For this review, take the finished solid that the model builds, in its own axes (mm). Face numbers are marked on the shaded views. A direction names the side the tool comes from. Give positions to 0.01 mm unless a question says otherwise; leave off trailing zeros. Order: outer loops, then holes, each group sorted by start corner. A loop starts at its lowest first (then second) coordinate and runs counter-clockwise, first axis right, second up. Notation, with made-up numbers: M -38,82.5 L -9,82.5 A31 ccw -9,112.5 Z; hole C 87,50 d8. An arc over 180 degrees is marked long. Answer as CSV lines item,"result". Start each with the question number.
1. We need section B-B, the plane z = -5. Give the boundary of the cut face in (x, y), and give its area (3 significant figures).
2. Machinability: for the marked faces 1 and 2, which of the approach directions +Z, -Z, +X, -X, +Y, -Y give a long, thin tool a straight path to every point of the face, cutting with its end or side? Answer none if there is none.
3. Clearance check with flat-ended pins moving along their axes: P1, Ø5, axis at x = 25, z = -5, coming from the +Y side; P2, Ø3, axis at y = 1, z = -2.5, coming from the -X side; P3, Ø1.8, axis at x = 3.5, z = -5.5, coming from the +Y side; P4, Ø3, axis at x = 15, z = -5.5, coming from the +Y side. State where each tip first meets the part, or that it passes through.
4. We need section A-A, the plane x = 25. Give the boundary of the cut face in (y, z).
5. Mouldability with a two-part tool opening along X and no side actions: class the marked faces 3, 4 and 5 as pulls with the +X half, pulls with the -X half, needs draft (parallel to the pull), parting line crosses it, or undercut.
6. For line 1 along X through (y, z) = (5.95, -5); line 2 along Z through (x, y) = (5, 5.95); line 3 along X through (y, z) = (6.25, -6.5), list the stretches that pass through material, from the lowest coordinate up.
7. We need section C-C, the plane x = 5. Give the boundary of the cut face in (y, z).
8. We need section D-D, the plane z = -7.5. Give the boundary of the cut face in (x, y).
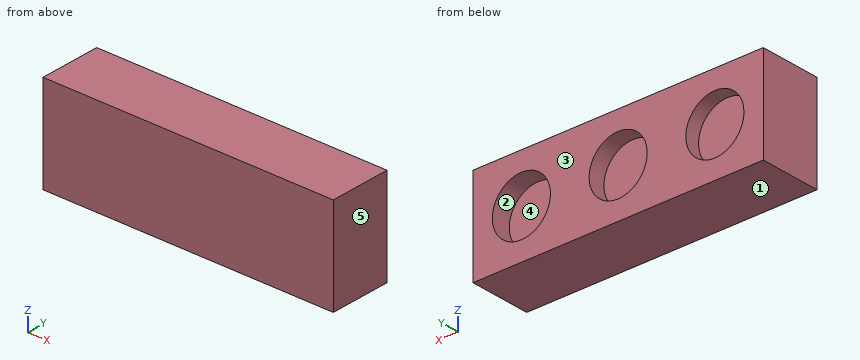
from build123d import *

# Parameters (mm, degrees)
SKETCH1_W           = 30
SKETCH1_H           = 10
BOSS_EXTRUDE1_DEPTH = 6.35
SKETCH2_R           = 3
CUT_EXTRUDE1_DEPTH  = 1.75
SKETCH4_R           = 3
CUT_EXTRUDE2_DEPTH  = 1.5
SKETCH5_R           = 3
CUT_EXTRUDE3_DEPTH  = 2


with BuildPart() as part:
    # Sketch1 → Boss-Extrude1 (new body)
    with BuildSketch(Plane(origin=(0, 0, 0), x_dir=(1, 0, 0), z_dir=(0, 1, 0))):
        with Locations((15, 5)):
            Rectangle(SKETCH1_W, SKETCH1_H)
    extrude(amount=BOSS_EXTRUDE1_DEPTH)

    # Sketch2 → Cut-Extrude1 (cut)
    with BuildSketch(Plane(origin=(0, 6.35, 0), x_dir=(1, 0, 0), z_dir=(0, 1, 0))):
        with Locations((15, 5)):
            Circle(SKETCH2_R)
    extrude(amount=-CUT_EXTRUDE1_DEPTH, mode=Mode.SUBTRACT)

    # Sketch4 → Cut-Extrude2 (cut)
    with BuildSketch(Plane(origin=(0, 6.35, 0), x_dir=(1, 0, 0), z_dir=(0, 1, 0))):
        with Locations((5, 5)):
            Circle(SKETCH4_R)
    extrude(amount=-CUT_EXTRUDE2_DEPTH, mode=Mode.SUBTRACT)

    # Sketch5 → Cut-Extrude3 (cut)
    with BuildSketch(Plane(origin=(0, 6.35, 0), x_dir=(1, 0, 0), z_dir=(0, 1, 0))):
        with Locations((25, 5)):
            Circle(SKETCH5_R)
    extrude(amount=-CUT_EXTRUDE3_DEPTH, mode=Mode.SUBTRACT)


solid = part.part
Result set:
1,outline,"M 0,0 L 30,0 L 30,6.35 L 28,6.35 L 28,4.35 L 22,4.35 L 22,6.35 L 18,6.35 L 18,4.6 L 12,4.6 L 12,6.35 L 8,6.35 L 8,4.85 L 2,4.85 L 2,6.35 L 0,6.35 Z"
1,area,"159 mm2"
2,face 1,"-Z, +X, -X, +Y, -Y"
2,face 2,"+Y"
3,P1,"y = 4.35"
3,P2,"x = 0"
3,P3,"y = 4.85"
3,P4,"y = 4.6"
4,outline,"M 0,-10 L 6.35,-10 L 6.35,-8 L 4.35,-8 L 4.35,-2 L 6.35,-2 L 6.35,0 L 0,0 Z"
5,face 3,"needs draft"
5,face 4,"undercut"
5,face 5,"pulls with the +X half"
6,line 1,"0 to 2, 8 to 12, 18 to 22, 28 to 30"
6,line 2,"-10 to -8, -2 to 0"
6,line 3,"0 to 2.4, 7.6 to 12.4, 17.6 to 22.4, 27.6 to 30"
7,outline,"M 0,-10 L 6.35,-10 L 6.35,-8 L 4.85,-8 L 4.85,-2 L 6.35,-2 L 6.35,0 L 0,0 Z"
8,outline,"M 0,0 L 30,0 L 30,6.35 L 26.66,6.35 L 26.66,4.35 L 23.34,4.35 L 23.34,6.35 L 16.66,6.35 L 16.66,4.6 L 13.34,4.6 L 13.34,6.35 L 6.66,6.35 L 6.66,4.85 L 3.34,4.85 L 3.34,6.35 L 0,6.35 Z"
